from build123d import *

# Parameters (mm, degrees)
SKETCH2_W           = 254
SKETCH2_H           = 254
BOSS_EXTRUDE1_DEPTH = 6.35
SKETCH3_R           = 3.25
CUT_EXTRUDE1_DEPTH  = 6.35


with BuildPart() as part:
    # Sketch2 → Boss-Extrude1 (new body)
    with BuildSketch(Plane.XY):
        with Locations((127, 127)):
            Rectangle(SKETCH2_W, SKETCH2_H)
    extrude(amount=BOSS_EXTRUDE1_DEPTH)

    # Sketch3 → Cut-Extrude1 (cut)
    with BuildSketch(Plane.XY.offset(6.35)):
        with Locations((71.12, 208.28)):
            Circle(SKETCH3_R)
        with Locations((182.88, 208.28)):
            Circle(SKETCH3_R)
        with Locations((182.88, 96.52)):
            Circle(SKETCH3_R)
        with Locations((71.12, 96.52)):
            Circle(SKETCH3_R)
        with BuildLine():
            Line((72.299743879, 196.579231637), (82.820768363, 207.100256121))
            ThreePointArc((82.820768363, 207.100256121), (86.940944893, 209.853270063), (91.801024484, 210.82))
            Line((91.801024484, 210.82), (162.198975516, 210.82))
            ThreePointArc((162.198975516, 210.82), (167.059055107, 209.853270063), (171.179231637, 207.100256121))
            Line((171.179231637, 207.100256121), (181.700256121, 196.579231637))
            ThreePointArc((181.700256121, 196.579231637), (184.453270063, 192.459055107), (185.42, 187.598975516))
            Line((185.42, 187.598975516), (185.42, 117.201024484))
            ThreePointArc((185.42, 117.201024484), (184.453270063, 112.340944893), (181.700256121, 108.220768363))
            Line((181.700256121, 108.220768363), (171.179231637, 97.699743879))
            ThreePointArc((171.179231637, 97.699743879), (167.059055107, 94.946729937), (162.198975516, 93.98))
            Line((162.198975516, 93.98), (91.801024484, 93.98))
            ThreePointArc((91.801024484, 93.98), (86.940944893, 94.946729937), (82.820768363, 97.699743879))
            Line((82.820768363, 97.699743879), (72.299743879, 108.220768363))
            ThreePointArc((72.299743879, 108.220768363), (69.546729937, 112.340944893), (68.58, 117.201024484))
            Line((68.58, 117.201024484), (68.58, 187.598975516))
            ThreePointArc((68.58, 187.598975516), (69.546729937, 192.459055107), (72.299743879, 196.579231637))
        make_face()
    extrude(amount=-CUT_EXTRUDE1_DEPTH, mode=Mode.SUBTRACT)


solid = part.part
Part model, mm, in its own coordinate system. A direction names the side the tool comes from. Coordinates: 2 decimals unless noted, no trailing zeros. Loops run counter-clockwise (first coordinate to the right, second up) from the corner with the lowest first, then second, coordinate; pieces in that order, holes last. Notation, with made-up numbers: (11, 36.25) -> (40, 36.25) arc R22 cw to (40, 59.25) -> close; hole circle Ø10 at (21, 24). An arc over 180 degrees is marked (long way). Use a Markdown table: item, result. Add a question column.
Item 1: Band-saw the part on A-A on y = 154.5. Write the cut outline in (x, z).
Item 2: Band-saw the part on C-C on x = 147.5. Write the cut outline in (y, z).
Item 3: Probe probe 1 along Y at (x, z) = (71.12, 3); probe 2 along X at (y, z) = (208.28, 3.75); probe 3 along Y at (x, z) = (139.5, 1.25). List the from-to ranges inside material, lowest first.
Item 4: Which spindle directions (+Z, -Z, +X, -X, +Y, -Y) get a long thin tool onto all of the face, cutting with end or side? Do faces 1 (the flat face through (77.63, 102.89, 3.22)), 2 (the flat face through (125, 254, 3)). Say none if no direction does.
Item 5: Band-saw the part on B-B on z = 4.5. Write the cut outline in (x, y).
Item 6: Pull direction X, two halves, no side cores. Call faces 3 (the cylindrical face through (86.88, 209.83, 3.22)), 4 (the flat face through (0, 125, 3)), 5 (the flat face through (125, 72, 0)): +X half, -X half, draft (parallel to the pull), parting line (faces both ways), or undercut.
Geometry says:
| question | item | result |
|---|---|---|
| 1 | outline | (0, 0) -> (68.58, 0) -> (68.58, 6.35) -> (0, 6.35) -> close; (185.42, 0) -> (254, 0) -> (254, 6.35) -> (185.42, 6.35) -> close |
| 2 | outline | (0, 0) -> (93.98, 0) -> (93.98, 6.35) -> (0, 6.35) -> close; (210.82, 0) -> (254, 0) -> (254, 6.35) -> (210.82, 6.35) -> close |
| 3 | probe 1 | 0 to 93.27, 99.77 to 109.58, 195.22 to 205.03, 211.53 to 254 |
| 3 | probe 2 | 0 to 67.87, 74.37 to 84.18, 169.82 to 179.63, 186.13 to 254 |
| 3 | probe 3 | 0 to 93.98, 210.82 to 254 |
| 4 | face 1 | +Z, -Z |
| 4 | face 2 | +Z, -Z, +X, -X, +Y |
| 5 | outline | (0, 0) -> (254, 0) -> (254, 254) -> (0, 254) -> close; hole circle Ø6.5 at (71.12, 96.52); hole circle Ø6.5 at (71.12, 208.28); hole (68.58, 117.2) arc R12.7 ccw to (72.3, 108.22) -> (82.82, 97.7) arc R12.7 ccw to (91.8, 93.98) -> (162.2, 93.98) arc R12.7 ccw to (171.18, 97.7) -> (181.7, 108.22) arc R12.7 ccw to (185.42, 117.2) -> (185.42, 187.6) arc R12.7 ccw to (181.7, 196.58) -> (171.18, 207.1) arc R12.7 ccw to (162.2, 210.82) -> (91.8, 210.82) arc R12.7 ccw to (82.82, 207.1) -> (72.3, 196.58) arc R12.7 ccw to (68.58, 187.6) -> close; hole circle Ø6.5 at (182.88, 96.52); hole circle Ø6.5 at (182.88, 208.28) |
| 6 | face 3 | undercut |
| 6 | face 4 | -X half |
| 6 | face 5 | draft |
